```python
from build123d import *

# Parameters (mm, degrees)
F0_R      = 15.5
F0_R_2    = 13.25
F1_DEPTH  = 90
F2_R      = 15.5
F3_DEPTH  = 2
F4_R      = 5
F5_DEPTH  = 90.001
F6_W      = 25
F6_H      = 75
F7_DEPTH  = 30
F9_DEPTH  = 6
F10_W     = 5.0829965621
F10_H     = 1.5
F11_DEPTH = 6
F13_DEPTH = 25
F15_DEPTH = 25
F16_DEPTH = 25


# Not quite as in the source:
# - a feature names something its author has since deleted; it is built from what else it names


with BuildPart() as f1:
    # F0 (on Top) → F1 (new body)
    with BuildSketch(Plane.XY):
        Circle(F0_R)
        Circle(F0_R_2, mode=Mode.SUBTRACT)
    extrude(amount=F1_DEPTH)

    # F2 (on Top) → F3 (join)
    with BuildSketch(Plane.XY):
        Circle(F2_R)
    extrude(amount=F3_DEPTH)

    # F4 (on Top) → F5 (cut, through all)
    with BuildSketch(Plane.XY):
        Circle(F4_R)
    extrude(amount=F5_DEPTH, mode=Mode.SUBTRACT)

    # F6 (on Front) → F7 (cut, symmetric)
    with BuildSketch(Plane.XZ):
        with Locations((3, 42.5)):
            Rectangle(F6_W, F6_H)
    extrude(amount=F7_DEPTH, both=True, mode=Mode.SUBTRACT)

    # F8 (on Front) → F9 (join, symmetric)
    with BuildSketch(Plane.XZ):
        with BuildLine():
            Line((-14.3252154812, 74.3832364678), (-15.3322340921, 74.3832364678))
            ThreePointArc((-15.3322340921, 74.3832364678), (-22.3824376382, 71.9712620232), (-24.7944127768, 64.9210587144))
            Line((-24.7944127768, 64.9210587144), (-24.7944127768, 16.9092640281))
            Line((-24.7944127768, 16.9092640281), (-19.7944119573, 16.9092640281))
            Line((-19.7944119573, 16.9092640281), (-19.7944119573, 65.3066100025))
            ThreePointArc((-19.7944119573, 65.3066100025), (-18.9325593375, 68.3469659349), (-15.9612301203, 69.4229570209))
            Line((-15.9612301203, 69.4229570209), (-14.3252154812, 69.4229570209))
            Line((-14.3252154812, 69.4229570209), (-14.3252154812, 74.3832364678))
        make_face()
    extrude(amount=F9_DEPTH, both=True)

    # F10 (on Front) → F11 (join, symmetric)
    with BuildSketch(Plane.XZ):
        with BuildLine():
            Line((-14.3252154812, 74.3832364678), (-15.3322340921, 74.3832364678))
            ThreePointArc((-15.3322340921, 74.3832364678), (-22.3824376382, 71.9712620232), (-24.7944127768, 64.9210587144))
            Line((-24.7944127768, 64.9210587144), (-24.7944127768, 16.9092640281))
            Line((-24.7944127768, 16.9092640281), (-19.7944119573, 16.9092640281))
            Line((-19.7944119573, 16.9092640281), (-19.7944119573, 18.4092640281))
            Line((-19.7944119573, 18.4092640281), (-19.7944119573, 65.3066100025))
            ThreePointArc((-19.7944119573, 65.3066100025), (-18.9325593375, 68.3469659349), (-15.9612301203, 69.4229570209))
            Line((-15.9612301203, 69.4229570209), (-14.3252154812, 69.4229570209))
            Line((-14.3252154812, 69.4229570209), (-14.3252154812, 74.3832364678))
        make_face()
        with Locations((-17.2529136762, 17.6592640281)):
            Rectangle(F10_W, F10_H)
    extrude(amount=F11_DEPTH, both=True)

    # F12 (on Top) → F13 (cut)
    with BuildSketch(Plane.XY):
        with BuildLine():
            Line((-13.8731463173, 7.0058838464), (-15.6120072238, 7.0058838464))
            ThreePointArc((-15.6120072238, 7.0058838464), (-17.1111072391, 0.1648850375), (-15.74411501, -6.7037318396))
            Line((-15.74411501, -6.7037318396), (-14.0216467162, -6.7037318396))
            ThreePointArc((-14.0216467162, -6.7037318396), (-15.5408577678, 0.1683361248), (-13.8731463173, 7.0058838464))
        make_face()
    extrude(amount=F13_DEPTH, mode=Mode.SUBTRACT)

    # F14 (on face) → F15 (cut)
    with BuildSketch(Plane.XY.offset(90)):
        with BuildLine():
            Line((11.193397513, 12.9792110231), (0, 0))
            Line((0, 0), (11.193397513, -12.9792110231))
            ThreePointArc((11.193397513, -12.9792110231), (17.1391967918, 0), (11.193397513, 12.9792110231))
        make_face()
    extrude(amount=-F15_DEPTH, mode=Mode.SUBTRACT)

    # F14 (on face) → F16 (cut)
    with BuildSketch(Plane.XY.offset(90)):
        with BuildLine():
            Line((10.1228583556, 11.7378762437), (8.6534111749, 10.0339909826))
            ThreePointArc((8.6534111749, 10.0339909826), (12.0461653249, 5.5183694119), (13.25, 0))
            ThreePointArc((13.25, 0), (12.0461653249, -5.5183694119), (8.6534111749, -10.0339909826))
            Line((8.6534111749, -10.0339909826), (10.1228583556, -11.7378762437))
            ThreePointArc((10.1228583556, -11.7378762437), (14.0917405687, -6.4554510102), (15.5, 0))
            ThreePointArc((15.5, 0), (14.0917405687, 6.4554510102), (10.1228583556, 11.7378762437))
        make_face()
        with BuildLine():
            Line((11.193397513, 12.9792110231), (10.1228583556, 11.7378762437))
            ThreePointArc((10.1228583556, 11.7378762437), (14.0917405687, 6.4554510102), (15.5, 0))
            ThreePointArc((15.5, 0), (14.0917405687, -6.4554510102), (10.1228583556, -11.7378762437))
            Line((10.1228583556, -11.7378762437), (11.193397513, -12.9792110231))
            ThreePointArc((11.193397513, -12.9792110231), (17.1391967918, 0), (11.193397513, 12.9792110231))
        make_face()
        with BuildLine():
            Line((8.6534111749, 10.0339909826), (0, 0))
            Line((0, 0), (8.6534111749, -10.0339909826))
            ThreePointArc((8.6534111749, -10.0339909826), (12.0461653249, -5.5183694119), (13.25, 0))
            ThreePointArc((13.25, 0), (12.0461653249, 5.5183694119), (8.6534111749, 10.0339909826))
        make_face()
    extrude(amount=-F16_DEPTH, mode=Mode.SUBTRACT)


solid = f1.part
```
Read the model definition and answer for the solid it produces. Units are mm, in the model's axes. A direction names the side the tool comes from. Give positions to 0.01 mm unless a question says otherwise; leave off trailing zeros. Write each loop counter-clockwise with the first axis right and the second up, starting at its lowest first coordinate (ties: lowest second). Pieces come first, ordered by that corner, then holes. Notation, with made-up numbers: M 63,-17 L 89,-17 A29 ccw 89,8 Z; hole C -28.5,-40 d7. An arc over 180 degrees is marked long. Put each result on its own line as item: value. Start each with the question number.
1. Consider line 1 along Y through (x, z) = (0, 0.45); line 2 along X through (y, z) = (0, 44); line 3 along Z through (x, y) = (-1.5, -8). Determine where each line is inside the solid, lowest interval first.
2. The part is cut by section B-B, the plane z = 47. Give the vertices of the cut face in (x, y).
3. For a pull along X with two mould halves and no side action, classify faces 6 (the flat face through (-15.7, -0.1, 69.423)), 7 (the flat face through (9.4, 10.9, 85.1)), 8 (the flat face through (0, -14, 80)), 9 (the flat face through (6, 0, 2)) as released by +X, released by -X, zero draft, split by the parting line, or undercut.
4. Each of these flat-tipped pins is pushed along its axis until it touches: pin 1 Ø3 at (x, y) = (-19, 1.5) entering from +Z; pin 2 Ø1 at (x, z) = (-10.5, 51) entering from -Y; pin 3 Ø2 at (x, z) = (-15, 30) entering from +Y. Where does it stop, or does it pass through?
5. Which of the six approach directions +Z, -Z, +X, -X, +Y, -Y give full straight-line access (tool end or side, diameter ignored) to faces 1 (the flat face through (0, 14, 80)), 2 (the flat face through (-24.794, 0, 41)), 3 (the flat face through (9.4, -10.9, 85.1)), 4 (the cylindrical face through (-13.237, 0.583, 55.162)), 5 (the flat face through (-18, 0, 18.409))?
6. The part is cut by section C-C, the plane y = 0. Give the vertices of the cut face in (x, z), and give its area (3 significant figures).
7. The part is cut by section A-A, the plane x = 0. Give the vertices of the cut face in (y, z).
8. The part is cut by section D-D, the plane x = -7. Give the vertices of the cut face in (y, z), and give its area (3 significant figures).
Final values:
1. line 1: y = -15.5 to -5, 5 to 15.5
1. line 2: x = -24.79 to -19.79, -15.5 to -13.25
1. line 3: z = 0 to 2
2. outline: M -24.79,-6 L -19.79,-6 L -19.79,6 L -24.79,6 Z; M -9.5,-12.25 L -9.5,-9.24 A13.25 cw -9.5,9.24 L -9.5,12.25 A15.5 ccw Z
3. face 6: undercut
3. face 7: released by +X
3. face 8: zero draft
3. face 9: undercut
4. pin 1: stops at z = 74.38
4. pin 2: stops at y = -11.84
4. pin 3: stops at y = 6.65
5. face 1: +X, +Y, -Y
5. face 2: -Z, -X, +Y, -Y
5. face 3: +Z, +X
5. face 4: +Z
5. face 5: +Y, -Y
6. outline: M -24.79,16.91 L -17.11,16.91 L -17.11,18.41 L -19.79,18.41 L -19.79,65.31 A3.46 cw -15.96,69.42 L -15.5,69.42 L -15.5,18.41 L -15.54,18.41 L -15.54,16.91 L -15.5,16.91 L -15.5,0 L -5,0 L -5,2 L -13.25,2 L -13.25,90 L -15.5,90 L -15.5,74.4 A8.46 ccw -24.79,64.92 Z; M 5,0 L 15.5,0 L 15.5,5 L 13.25,5 L 13.25,2 L 5,2 Z
6. area: 548 mm²
7. outline: M -15.5,0 L -5,0 L -5,2 L -13.25,2 L -13.25,5 L -15.5,5 Z; M -15.5,80 L -13.25,80 L -13.25,90 L -15.5,90 Z; M 5,0 L 15.5,0 L 15.5,5 L 13.25,5 L 13.25,2 L 5,2 Z; M 13.25,80 L 15.5,80 L 15.5,90 L 13.25,90 Z
8. outline: M -13.83,0 L 13.83,0 L 13.83,5 L 11.25,5 L 11.25,2 L -11.25,2 L -11.25,5 L -13.83,5 Z; M -13.83,80 L -11.25,80 L -11.25,90 L -13.83,90 Z; M 11.25,80 L 13.83,80 L 13.83,90 L 11.25,90 Z
8. area: 122 mm²
